Input: part model. Units: mm. Frame: model coordinates. A direction names the side the tool comes from. Round coordinates to 2 decimals unless told otherwise and drop trailing zeros. Order: outer loops, then holes, each group sorted by start corner. A loop starts at its lowest first (then second) coordinate and runs counter-clockwise, first axis right, second up. Notation, with made-up numbers: (-40, -0.75) -> (-8, -0.75) arc R13 ccw to (-8, 14.25) -> close; hole circle Ø4 at (14, 3.25). An arc over 180 degrees is marked (long way). Answer as CSV lines item,"result". Start each with the question number.
1) Section query C-C, the plane y = -1.5. Output: boundary loops of the cut face in (x, z).
2) Access query for faces 1 (the face through (-0.1, 3.3, 1.2)), 2 (the face through (0, -9, 0)), 3 (the face through (2.2, 2.5, -1.2)). Directions: +Z, -Z, +X, -X, +Y, -Y. A direction counts if a zero-diameter tool reaches every point of the face in a straight line with its end or side. Return the directions, or none.
3) Mould query, pull axis Z, two halves, no side actions, for faces 4 (the face through (-1.5, -13.06, 0.07)), 5 (the face through (0, -17, -2)), 6 (the face through (0.046, -5.521, -2.078)). Classes: +Z half, -Z half, draft (parallel to the pull), parting line (faces both ways), or undercut.
4) Section query D-D, the plane x = -2. Output: boundary loops of the cut face in (y, z), and give its area (3 significant figures).
5) Line query: L1, parallel to Z at x = 0, y = -14.75; L2, parallel to Y at x = -2.5, z = 0.75; L3, parallel to Z at x = 3, y = 2.75. Output: solid intervals per line, ascending.
6) Section query A-A, the plane z = 0. Output: boundary loops of the cut face in (x, y).
7) Section query B-B, the plane x = -3. Output: boundary loops of the cut face in (y, z).
8) First-contact query: P1, Ø5, axis at x = -0.5, y = -14.5, coming from the +Z side; P2, Ø1.5, axis at x = -3, z = -1, coming from the +Y side; P3, Ø3, axis at x = 2, y = -13, coming from the -Z side; P4, Ø0.9, axis at x = 0.5, z = 0.5, coming from the -Y side. Flat tips, straight axial feed; report the tip coordinate or a pass-through.
```python
from build123d import *

# Parameters (mm, degrees)
F2_R          = 3.5
F3_DEPTH      = 17
F7_DEPTH      = 6
F7_DEPTH_BACK = 6
F8_R          = 1.5
F9_DEPTH      = 8


with BuildPart() as f1:
    # F0 (on Right) → F1 (revolve)
    with BuildSketch(Plane.YZ):
        with BuildLine():
            Line((0, 5), (0, -5))
            ThreePointArc((0, -5), (5, 0), (0, 5))
        make_face()
    revolve(axis=Axis((0, 0, 0), (0, 0, -1)))

    # F2 (on Front) → F3 (join)
    with BuildSketch(Plane.XZ):
        Circle(F2_R)
    extrude(amount=F3_DEPTH)

    # F4 (on Right) → F5 (revolve, cut)
    with BuildSketch(Plane.YZ):
        with BuildLine():
            Line((0, 3.25), (0, -3.25))
            ThreePointArc((0, -3.25), (3.25, 0), (0, 3.25))
        make_face()
    revolve(axis=Axis((0, 0, 0), (0, 0, -1)), mode=Mode.SUBTRACT)

    # F6 (on Right) → F7 (cut, two sides)
    with BuildSketch(Plane.YZ) as f7_sk:
        Polygon((-4, 1.2), (5.5, 1.2), (5.5, 5.2), (-10.9282032303, 5.2), align=None)
        Polygon((-10.9282032303, -5.2), (5.5, -5.2), (5.5, -1.2), (-4, -1.2), align=None)
    extrude(amount=-F7_DEPTH, mode=Mode.SUBTRACT)
    extrude(f7_sk.sketch, amount=F7_DEPTH_BACK, mode=Mode.SUBTRACT)

    # F8 (on face) → F9 (cut)
    with BuildSketch(Plane.XZ.offset(17)):
        Circle(F8_R)
    extrude(amount=-F9_DEPTH, mode=Mode.SUBTRACT)


solid = f1.part
```
Findings:
1,outline,"(-4.62, -1.2) -> (-2.62, -1.2) arc R2.88 cw to (-2.62, 1.2) -> (-4.62, 1.2) arc R4.77 ccw to start; (2.62, -1.2) -> (4.62, -1.2) arc R4.77 ccw to (4.62, 1.2) -> (2.62, 1.2) arc R2.88 cw to start"
2,face 1,"+Z, +X, -X, +Y"
2,face 2,"-Y"
2,face 3,"-Z, +X, -X, +Y"
3,face 4,"undercut"
3,face 5,"draft"
3,face 6,"-Z half"
4,outline,"(-17, -2.87) -> (-6.9, -2.87) -> (-4, -1.2) -> (-2.26, -1.2) arc R2.56 cw to (-2.26, 1.2) -> (-4, 1.2) -> (-6.9, 2.87) -> (-17, 2.87) -> close; (2.26, -1.2) -> (4.42, -1.2) arc R4.58 ccw to (4.42, 1.2) -> (2.26, 1.2) arc R2.56 cw to start"
4,area,"78.5 mm^2"
5,L1,"z = -3.5 to -1.5, 1.5 to 3.5"
5,L2,"y = -17 to -1.94, 1.94 to 4.26"
5,L3,"z = -1.2 to 1.2"
6,outline,"(-3.5, -17) -> (-1.5, -17) -> (-1.5, -9) -> (1.5, -9) -> (1.5, -17) -> (3.5, -17) -> (3.5, -3.57) arc R5 ccw (long way) to (-3.5, -3.57) -> close; hole circle Ø6.5 at (0, 0)"
7,outline,"(-17, -1.8) -> (-5.04, -1.8) -> (-4, -1.2) -> (-0.35, -1.2) arc R1.25 cw to (-0.35, 1.2) -> (-4, 1.2) -> (-5.04, 1.8) -> (-17, 1.8) -> close; (0.35, -1.2) -> (3.82, -1.2) arc R4 ccw to (3.82, 1.2) -> (0.35, 1.2) arc R1.25 cw to start"
8,P1,"stops at z = 3.5"
8,P2,"stops at y = 4.38"
8,P3,"stops at z = -3.46"
8,P4,"stops at y = -9"
